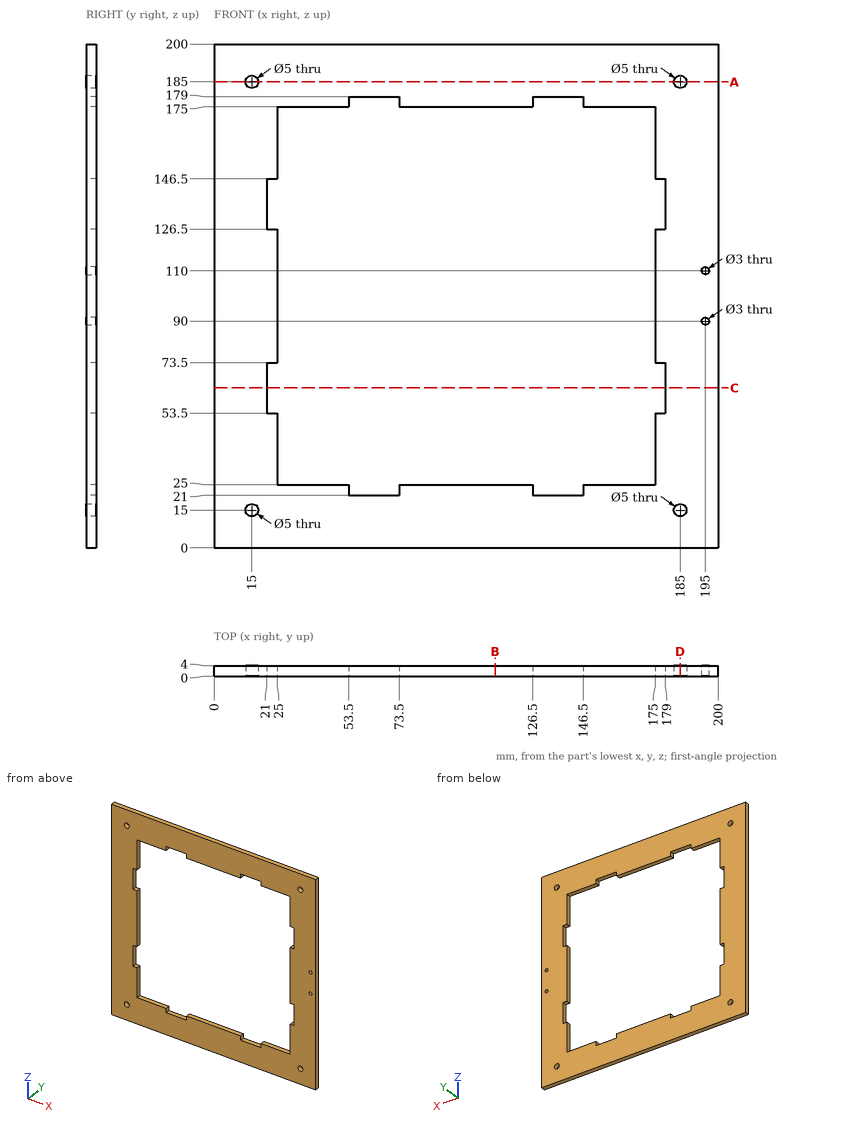
Verification items for this drawing (mm, ordinates from the low corner). Coordinates: 2 decimals unless noted, no trailing zeros. Order: outer loops, then holes, each group sorted by start corner. A loop starts at its lowest first (then second) coordinate and runs counter-clockwise, first axis right, second up.
Q1. Sectioned sample at C-C on z = 63.5. Record the cut outline in (x, y).
Reply:
outline: (0, 0) - (21, 0) - (21, 4) - (0, 4) - close; (179, 0) - (200, 0) - (200, 4) - (179, 4) - close
Q2. Sectioned sample at A-A on z = 185. Record the cut outline in (x, y).
Reply:
outline: (0, 0) - (12.5, 0) - (12.5, 4) - (0, 4) - close; (17.5, 0) - (182.5, 0) - (182.5, 4) - (17.5, 4) - close; (187.5, 0) - (200, 0) - (200, 4) - (187.5, 4) - close
Q3. Thickness scan on probe 1 along X at (y, z) = (2.9, 185); probe 2 along Z at (x, y) = (195, 1.5); probe 3 along X at (y, z) = (2.05, 110). Record the ranges inside material, lowest first.
Reply:
probe 1: x = 0 to 12.5, 17.5 to 182.5, 187.5 to 200
probe 2: z = 0 to 88.5, 91.5 to 108.5, 111.5 to 200
probe 3: x = 0 to 25, 175 to 193.5, 196.5 to 200
Q4. Sectioned sample at D-D on x = 185. Record the cut outline in (y, z), and give its area (3 significant figures).
Reply:
outline: (0, 0) - (4, 0) - (4, 12.5) - (0, 12.5) - close; (0, 17.5) - (4, 17.5) - (4, 182.5) - (0, 182.5) - close; (0, 187.5) - (4, 187.5) - (4, 200) - (0, 200) - close
area: 760 mm2
Q5. Depth check by flat-ended pin: pin 1 Ø4.5 at (x, z) = (15, 185) entering from +Y. Enter the tip coordinate at first touch or a pass-through.
Reply:
pin 1: passes through
Q6. Sectioned sample at B-B on x = 111.5. Record the cut outline in (y, z).
Reply:
outline: (0, 0) - (4, 0) - (4, 25) - (0, 25) - close; (0, 175) - (4, 175) - (4, 200) - (0, 200) - close
